Read the model definition and answer for the solid it produces. Units are mm, in the model's axes. A direction names the side the tool comes from. Round coordinates to 2 decimals unless told otherwise and drop trailing zeros. Loops run counter-clockwise (first coordinate to the right, second up) from the corner with the lowest first, then second, coordinate; pieces in that order, holes last. Notation, with made-up numbers: M 79,12 L 124,12 A20 cw 124,29 Z; hole C 8.5,63 d9. An arc over 180 degrees is marked long. Answer as CSV lines item,"result".
Autodesk Inventor part; units mm, degrees
ref_plane "YZ Plane" through (0, 0, 0) normal (1, 0, 0) x (0, 1, 0)
ref_plane "XZ Plane" through (0, 0, 0) normal (0, 1, 0) x (-1, 0, 0)
ref_plane "XY Plane" through (0, 0, 0) normal (0, 0, 1) x (1, 0, 0)
sketch "Sketch1" plane through (0, 0, 0) normal (0, 0, 1) x (1, 0, 0)
  line L0 (-84.0821, 192.7052) -> (642.9929, 192.7052)
  line L1 (642.9929, 192.7052) -> (642.9929, -137.4948)
  line L2 (642.9929, -137.4948) -> (-84.0821, -137.4948)
  line L3 (-84.0821, -137.4948) -> (-84.0821, 192.7052)
  circle A0 centre (131.8179, -91.7748) radius 4.7625
  circle A1 centre (318.0537, 116.5052) radius 12.7
  line L4 (642.9929, -137.4948) -> (592.1929, -137.4948)
  line L5 (592.1929, -137.4948) -> (592.1929, -73.9948)
  line L6 (592.1929, -73.9948) -> (642.9929, -73.9948)
  line L7 (642.9929, -73.9948) -> (642.9929, -137.4948)
  line L8 (642.9929, 192.7052) -> (592.6352, 192.7052)
  line L9 (642.9929, 2.2052) -> (642.9929, 192.7052)
  line L10 (-84.0821, 53.0052) -> (5.7204, 53.0052) construction
  line L11 (-84.0821, 65.7052) -> (68.3179, -137.4948)
  line L12 (595.3679, 192.7052) -> (595.3679, 2.2052)
  line L13 (595.3679, 2.2052) -> (642.9929, 2.2052)
  point P0 (0, 0)
  dimension "d0" = 727.075
  dimension "d2" = 9.525
  dimension "d3" = 25.4
  dimension "d4" = 215.9
  dimension "d5" = 279.4
  dimension "d14" = 152.4
  dimension "d15" = 203.2
  dimension "d16" = 330.2
  dimension "d17" = 63.5
  dimension "d19" = 50.8
  dimension "d20" = 139.7
  dimension "d21" = 45.72
  dimension "d22" = 254
extrude "Extrusion1" add sketch "Sketch1" along normal blind 9.525 contours L0 L12 L13 L1 L6 L5 L2 L11 L3
sketch "Sketch2" plane through (0, 0, 9.525) normal (0, 0, 1) x (1, 0, 0)
  line L0 (595.3679, 2.2052) -> (595.3679, 192.7052)
  line L1 (595.3679, 192.7052) -> (-84.0821, 192.7052)
  line L2 (-84.0821, 192.7052) -> (-84.0821, 65.7052)
  line L3 (68.3179, -137.4948) -> (592.1929, -137.4948)
  line L4 (592.1929, -137.4948) -> (592.1929, -73.9948)
  line L5 (-84.0821, 127.1732) -> (106.4179, 192.7052)
  line L6 (379.4679, 192.7052) -> (646.1679, 59.3552)
  line L7 (595.3679, 84.7552) -> (595.3679, 192.7052)
  point P0 (0, 0)
  dimension "d25" = 190.5
  dimension "d26" = 61.468
  dimension "d28" = 196.85
  dimension "d30" = 53.975
  dimension "d31" = 212.725
extrude "Extrusion2" cut sketch "Sketch2" against normal blind 25.4
sketch "Sketch3" plane through (0, 0, 9.525) normal (0, 0, 1) x (1, 0, 0)
  line L0 (592.1929, -137.4948) -> (740.2432, -137.4948)
  line L1 (740.2432, -137.4948) -> (740.2432, 103.8052)
  line L2 (740.2432, 103.8052) -> (592.1929, 103.8052)
  line L3 (592.1929, 103.8052) -> (592.1929, -137.4948)
  point P0 (0, 0)
extrude "Extrusion3" cut sketch "Sketch3" against normal blind 25.4
sketch "Sketch4" plane through (0, 0, 9.525) normal (0, 0, 1) x (1, 0, 0)
  line L0 (592.1929, -137.4948) -> (592.1929, 86.3427)
  line L1 (592.1929, 86.3427) -> (379.4679, 192.7052)
  line L2 (68.3179, -137.4948) -> (592.1929, -137.4948)
  line L3 (592.1929, 86.3427) -> (646.1679, 59.3552)
  line L4 (646.1679, 59.3552) -> (646.1679, 40.3052)
  line L5 (646.1679, 40.3052) -> (592.1929, 40.3052)
  point P0 (0, 0)
  dimension "d37" = 53.975
  dimension "d38" = 19.05
extrude "Extrusion4" add sketch "Sketch4" against normal blind 9.525
sketch "Sketch5" plane through (0, 0, 9.525) normal (0, 0, 1) x (1, 0, 0)
  line L0 (592.1929, 40.3052) -> (646.1679, 40.3052)
  line L1 (646.1679, 40.3052) -> (646.1679, 5.3802)
  line L2 (646.1679, 5.3802) -> (592.1929, 5.3802)
  line L3 (592.1929, 5.3802) -> (592.1929, 40.3052)
  point P0 (0, 0)
  dimension "d41" = 34.925
extrude "Extrusion5" add sketch "Sketch5" against normal blind 9.525
sketch "Sketch6" plane through (0, 0, 9.525) normal (0, 0, 1) x (1, 0, 0)
  line L0 (-84.0821, 65.7052) -> (68.3179, -137.4948)
  line L1 (68.3179, -137.4948) -> (592.1929, -137.4948)
  line L2 (592.1929, -137.4948) -> (592.1929, 40.3052)
  line L3 (147.7945, 9.1902) -> (225.2645, 9.1902)
  line L4 (341.7489, -137.4948) -> (170.3104, -117.1748)
  line L5 (170.3104, -117.1748) -> (53.0779, -117.1748)
  line L6 (68.3179, -137.4948) -> (592.1929, -137.4948)
  line L7 (592.1929, -96.6594) -> (439.7929, -137.4948)
  line L8 (439.7929, -137.4948) -> (592.1929, -137.4948)
  line L9 (592.1929, -137.4948) -> (592.1929, -96.6594)
  point P0 (0, 0)
  point P1 (0, 0)
  dimension "d47" = 20.32
  dimension "d50" = 152.4
  dimension "d53" = 173.24
  dimension "d54" = 165
  dimension "d55" = 98.044
extrude "Extrusion7" cut sketch "Sketch6" against normal blind 25.4
sketch "Sketch7" plane through (0, 0, 0) normal (0, 0, -1) x (-1, 0, 0)
  line L0 (-68.3179, -137.4948) -> (-592.1929, -137.4948)
  line L1 (84.0821, 192.7052) -> (84.0821, 65.7052)
  circle A0 centre (-147.7945, -23.1948) radius 32.385
  circle A1 centre (-225.2645, -23.1948) radius 32.385
  line L2 (-225.2645, 9.1902) -> (-147.7945, 9.1902)
  line L3 (-225.2645, -55.5798) -> (-147.7945, -55.5798)
  circle A2 centre (-323.5837, 116.5052) radius 12.7
  line L4 (-595.3679, 192.7052) -> (-595.3679, 2.2052)
  line L5 (-595.3679, 2.2052) -> (-642.9929, 2.2052)
  line L6 (-642.9929, -73.9948) -> (-642.9929, 2.2052)
  line L7 (-642.9929, -73.9948) -> (-592.1929, -73.9948)
  line L8 (-592.1929, -73.9948) -> (-592.1929, -137.4948)
  line L9 (84.0821, 65.7052) -> (-68.3179, -137.4948)
  line L10 (-595.3679, 192.7052) -> (84.0821, 192.7052)
  circle A3 centre (-131.8179, -86.6948) radius 4.7625
  point P0 (0, 0)
  point P1 (0, 0)
  dimension "d56" = 64.77
  dimension "d57" = 231.8766
  dimension "d58" = 114.3
  dimension "d59" = 64.77
  dimension "d60" = 77.47
extrude "Extrusion8" cut sketch "Sketch7" against normal blind 25.4 contours A0 | A0 L3 A1 L2 | A1
sketch "Sketch8" plane through (0, 0, 9.525) normal (0, 0, 1) x (1, 0, 0)
  line L0 (-84.0821, 65.7052) -> (53.0779, -117.1748)
  line L1 (-84.0821, 127.1732) -> (-84.0821, 65.7052)
  line L2 (53.0779, -117.1748) -> (170.3104, -117.1748)
  arc A0 (82.3351, -98.9312) -> (-55.5071, 27.6052) centre (-44.6649, -98.9312) ccw
  line L3 (341.7489, -137.4948) -> (439.7929, -137.4948)
  line L4 (82.3351, -117.1748) -> (82.3351, -74.3195)
  point P0 (0, 0)
  point P1 (81.0179, -117.1748)
  dimension "d65" = 38.1
  dimension "d68" = 127
  dimension "d69" = 165.1
extrude "Extrusion9" cut sketch "Sketch8" against normal blind 25.4
sketch "Sketch12" plane through (0, 0, 9.525) normal (0, 0, 1) x (1, 0, 0)
  line L0 (341.7489, -137.4948) -> (439.7929, -137.4948)
  line L1 (439.7929, -137.4948) -> (592.1929, -96.6594)
  line L2 (592.1929, -96.6594) -> (592.1929, 5.3802)
  line L3 (439.7929, -137.4948) -> (592.1929, -79.2096)
  point P0 (341.4151, -137.4948)
  point P1 (0, 0)
  dimension "d85" = 17.4498
extrude "Extrusion13" cut sketch "Sketch12" against normal blind 9.525
sketch "Sketch16" plane through (0, 0, 9.525) normal (0, 0, 1) x (1, 0, 0)
  circle A0 centre (131.8179, -91.7748) radius 4.7625
  line L0 (82.3351, -117.1748) -> (170.3104, -117.1748)
  line L1 (170.3104, -117.1748) -> (341.7489, -137.4948)
  line L2 (341.7489, -137.4948) -> (439.7929, -137.4948)
  circle A1 centre (131.8179, -91.7748) radius 38.1
  line L3 (131.8179, -129.8748) -> (82.3351, -129.8748)
  line L4 (82.3351, -129.8748) -> (277.4594, -129.8748)
  line L5 (82.3351, -129.8748) -> (82.3351, -117.1748)
  point P0 (0, 0)
  dimension "d108" = 76.2
extrude "Extrusion18" add sketch "Sketch16" against normal blind 9.525 contours L0 A1 L3 L5 | L0 A1 | L0 L1 L4 A1 picked at (139.3083, -118.9641)
sketch "Sketch17" plane through (0, 0, 9.525) normal (0, 0, 1) x (1, 0, 0)
  line L0 (82.3351, -98.9312) -> (82.3351, -129.8748)
  line L1 (82.3351, -129.8748) -> (277.4594, -129.8748)
  line L2 (277.4594, -129.8748) -> (341.7489, -137.4948)
  line L3 (341.7489, -137.4948) -> (236.6401, -107.9038)
  line L4 (236.6401, -107.9038) -> (142.6601, -129.8748)
  point P0 (0, 0)
  dimension "d111" = 154.305
  dimension "d112" = 21.971
  dimension "d115" = 60.325
extrude "Extrusion19" cut sketch "Sketch17" against normal blind 9.525
sketch "Sketch18" plane through (0, 0, 9.525) normal (0, 0, 1) x (1, 0, 0)
  line L0 (-84.0821, 65.7052) -> (-55.5071, 27.6052)
  arc A0 (82.3351, -98.9312) -> (-55.5071, 27.6052) centre (-44.6649, -98.9312) ccw
  line L1 (-84.0821, 65.7052) -> (-45.0245, 28.0683)
  point P0 (0, 0)
extrude "Extrusion20" cut sketch "Sketch18" against normal blind 9.525
properties part number "ShooterMountRight_NERDS"
1) Straight lines are drawn through the part: line 1 (Y direction, x = 144, z = 4.5); line 2 (Y direction, x = 310, z = 3); line 3 (Y direction, x = 459, z = 2). For each, find the intervals that lie inside material, in ascending order.
Evaluation:
line 1,"y = -129.56 to -55.36, 8.97 to 192.71"
line 2,"y = -128.56 to 106.69, 126.32 to 192.71"
line 3,"y = -130.15 to 152.94"
2) Find section A-A, the plane y = -10. Give the vertices of the cut face in (x, z) (3 decimals).
Evaluation:
outline,"M 46.001,0 L 118.219,0 L 118.219,9.525 L 46.001,9.525 Z; M 254.84,0 L 592.193,0 L 592.193,9.525 L 254.84,9.525 Z"
3) Each of these flat-tipped pins is pushed along its axis until it touches: P1, Ø1, axis at x = 216.5, z = 7.5, coming from the -Y side; P2, Ø3, axis at x = 204.5, z = 4.5, coming from the -Y side; P3, Ø5, axis at y = -112.5, z = 5.5, coming from the -X side. Where does it stop, or does it pass through?
Evaluation:
P1,"stops at y = -112.73"
P2,"stops at y = -115.77"
P3,"stops at x = 82.34"
4) Determine the mould class of faces 4 (the flat face through (9.83, 159.48, 4.83)), 5 (the flat face through (276, 30, 9.525)), 6 (the cylindrical face through (115.417, -23.907, 4.696)) for opening direction X: released by +X, released by -X, zero draft, split by the parting line, or undercut.
Evaluation:
face 4,"released by -X"
face 5,"zero draft"
face 6,"undercut"
5) Find section B-B, the plane z = 1.75. Give the vertices of the cut face in (x, y) (1 decimal), then the cut area to 3 significant figures.
Evaluation:
outline,"M -84.1,65.7 L -45,28.1 A127 cw 82.3,-98.9 L 82.3,-129.9 L 142.7,-129.9 L 236.6,-107.9 L 341.7,-137.5 L 439.8,-137.5 L 592.2,-79.2 L 592.2,5.4 L 646.2,5.4 L 646.2,59.4 L 379.5,192.7 L 106.4,192.7 L -84.1,127.2 Z; hole C 131.8,-91.8 d9.5; hole M 147.8,-55.6 L 225.3,-55.6 A32.4 ccw 225.3,9.2 L 147.8,9.2 A32.4 ccw Z; hole C 318.1,116.5 d25.4"
area,"167,000 mm^2"
6) Find section D-D, the plane y = -44.5. Give the vertices of the cut face in (x, z) (3 decimals), then the cut area to 3 significant figures.
Evaluation:
outline,"M 70.079,0 L 123.404,0 L 123.404,9.525 L 70.079,9.525 Z; M 249.655,0 L 592.193,0 L 592.193,9.525 L 249.655,9.525 Z"
area,"3,770 mm^2"
7) A tool of negligible diameter and unlimited length cuts with its end or side. For faces 1 (the flat face through (276, 30, 0)), 2 (the cylindrical face through (257.64, -22.48, 4.7)), 3 (the flat face through (190.308, -118.736, 4.829)), from which of +Z, -Z, +X, -X, +Y, -Y can it reach the whole face along a straight path? Write none if from no direction.
Evaluation:
face 1,"-Z, +X, -X, +Y, -Y"
face 2,"+Z, -Z"
face 3,"+Z, -Z, -Y"
8) Find section C-C, the plane x = 497. Give the vertices of the cut face in (y, z) (3 decimals).
Evaluation:
outline,"M -115.616,0 L 133.939,0 L 133.939,9.525 L -115.616,9.525 Z"
